```python
from build123d import *

# Parameters (mm, degrees)
CHAMFER1_SIZE      = 0.5
CUT_EXTRUDE1_START = -15
CUT_EXTRUDE1_DEPTH = 15
SKETCH3_R          = 0.75
CUT_EXTRUDE2_DEPTH = 86.691656537


with BuildPart() as part:
    # Sketch1 → Revolve1 (revolve)
    with BuildSketch(Plane(origin=(0, 0, 0), x_dir=(0, 0, -1), z_dir=(1, 0, 0))):
        Polygon((0, -40.8), (0, 40.8), (4, 40.8), (4, 19.2), (18.5, 19.2), (18.5, -38.8), (4, -38.8), (4, -40.8), align=None)
    revolve(axis=Axis((0, -40.8, 0), (0, 1, 0)))

    # Chamfer1
    chamfer1_edges = [part.edges().sort_by_distance(p)[0] for p in [
        (0, 40.8, 4),
    ]]
    chamfer(chamfer1_edges, length=CHAMFER1_SIZE)

    # Sketch2 → Cut-Extrude1 (cut)
    with BuildSketch(Plane(origin=(0, 40.8, 0), x_dir=(1, 0, 0), z_dir=(0, 1, 0)).offset(CUT_EXTRUDE1_START)):
        with BuildLine():
            Line((-3.551675661, 1.84), (3.551675661, 1.84))
            ThreePointArc((3.551675661, 1.84), (0, 4), (-3.551675661, 1.84))
        make_face()
    extrude(amount=CUT_EXTRUDE1_DEPTH, mode=Mode.SUBTRACT)

    # Sketch3 → Cut-Extrude2 (cut, through all)
    with BuildSketch(Plane(origin=(0, 40.8, 0), x_dir=(1, 0, 0), z_dir=(0, 1, 0))):
        with Locations(Location((0, 0, 0), (0, 0, 270))):
            Circle(SKETCH3_R)
    extrude(amount=-CUT_EXTRUDE2_DEPTH, mode=Mode.SUBTRACT)


solid = part.part
```
Part model, mm, in its own coordinate system. A direction names the side the tool comes from. Round coordinates to 2 decimals unless told otherwise and drop trailing zeros. Order: outer loops, then holes, each group sorted by start corner. A loop starts at its lowest first (then second) coordinate and runs counter-clockwise, first axis right, second up. Notation, with made-up numbers: M 70.5,56 L 100.5,56 A14 ccw 100.5,76 Z; hole C 48,8 d5. An arc over 180 degrees is marked long. Answer in a Markdown table with one row per item. Add a question column.
Q1. Wall check: L1, parallel to X at y = 2, z = 0; L2, parallel to Y at x = 8, z = -10.5; L3, parallel to X at y = -5, z = -0.5. Give the ranges that are in metal, low to high. Write a range as from..to.
Q2. Mould opens along Z. For faces 1 (the face through (-4.4, -38.8, 0.3)), 2 (the face through (0, 33, -1.84)), 3 (the face through (0.225, 0.571, 0.715)) say: +Z half, -Z half, draft (parallel to the pull), parting line (faces both ways), or undercut.
Q3. Pin check, flat tips, straight feed: pin 1 (1.5 mm diameter, centred on y = 9.5, z = 6.5, fed in from -X); pin 2 (10 mm diameter, centred on x = -12, y = -21.5, fed in from -Z); pin 3 (1.5 mm diameter, centred on x = -6, z = -8, fed in from -Y); pin 4 (0.9 mm diameter, centred on x = 0, z = 0, fed in from +Y). Stop position of each tip, or through.
Q4. Cut at A-A on y = 33.5. Give the cut face in (x, z).
Q5. Cut at C-C on z = 7. Give the cut face in (x, y).
Q6. Cut at B-B on y = -17. Give the cut face in (x, z).
Q7. Cut at D-D on x = 12. Give the cut face in (y, z).
Q8. 3-axis set-ups, long thin cutter, end or side, ignore diameter. For faces 4 (the face through (3.905, -39.814, 0.867)), 5 (the face through (0, 27, 4)), 6 (the face through (18.06, -10.21, 4.01)), 7 (the face through (0, 25.8, -3)), 8 (the face through (1, -40.8, 0)): which of +Z, -Z, +X, -X, +Y, -Y reach the whole face in a straight line?
Established:
| question | item | result |
|---|---|---|
| 1 | L1 | x = -18.5..-0.75, 0.75..18.5 |
| 1 | L2 | y = -38.8..19.2 |
| 1 | L3 | x = -18.49..-0.56, 0.56..18.49 |
| 2 | face 1 | draft |
| 2 | face 2 | -Z half |
| 2 | face 3 | undercut |
| 3 | pin 1 | stops at x = -17.58 |
| 3 | pin 2 | stops at z = -17.12 |
| 3 | pin 3 | stops at y = -38.8 |
| 3 | pin 4 | passes through |
| 4 | outline | M -3.55,-1.84 L 3.55,-1.84 A4 ccw long Z; hole C 0,0 d1.5 |
| 5 | outline | M -17.12,-38.8 L 17.12,-38.8 L 17.12,19.2 L -17.12,19.2 Z |
| 6 | outline | C 0,0 d37; hole C 0,0 d1.5 |
| 7 | outline | M -38.8,-14.08 L 19.2,-14.08 L 19.2,14.08 L -38.8,14.08 Z |
| 8 | face 4 | -Y |
| 8 | face 5 | +Y |
| 8 | face 6 | +Y, -Y |
| 8 | face 7 | -Z, +X, -X, +Y |
| 8 | face 8 | +Z, -Z, +X, -X, -Y |
